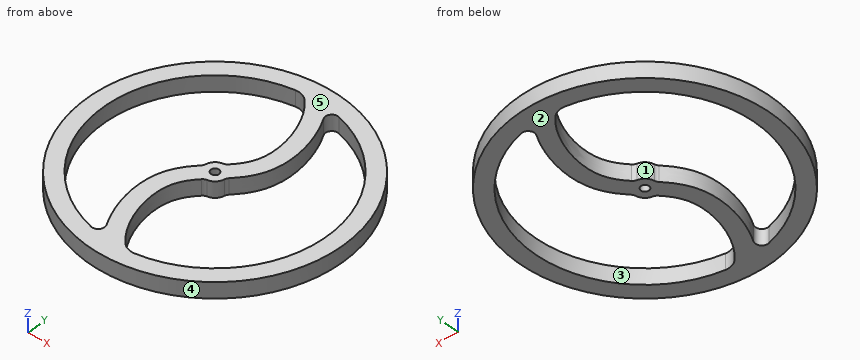
```python
from build123d import *

# Parameters (mm, degrees)
ESQUISSE1_R                  = 400
ESQUISSE1_R_2                = 350
BOSS_EXTRU_1_DEPTH           = 50
EXTRU_MINCE1_START           = -50
EXTRU_MINCE1_DEPTH           = 50
BOSS_EXTRU_2_START           = -50
BOSS_EXTRU_2_DEPTH           = 50
ENL_V_MAT_EXTRU_1_DEPTH      = 568.89083473
ENL_V_MAT_EXTRU_1_DEPTH_BACK = 568.89083473
ESQUISSE4_R                  = 12.5
ESQUISSE5_R                  = 35
ESQUISSE5_R_2                = 12.5
BOSS_EXTRU_3_DEPTH           = 50
CONG_2_R                     = 20


# Read off the part's stored shape, not the designer's step: Extru.-Mince1
with BuildPart() as part:
    # Esquisse1 → Boss.-Extru.1 (new body)
    with BuildSketch(Plane.XY):
        Circle(ESQUISSE1_R)
        Circle(ESQUISSE1_R_2, mode=Mode.SUBTRACT)
    extrude(amount=BOSS_EXTRU_1_DEPTH)

    # Extru.-Mince1 outline → Extru.-Mince1 (add)
    with BuildSketch(Plane.XY.offset(50).offset(EXTRU_MINCE1_START)):
        with BuildLine():
            add(Edge.make_bspline(
                [(-17.578582702, 332.223795956), (-13.006029397, 327.702076571), (-8.525799104, 322.703406145), (0.139661855, 311.878345733), (4.324902329, 306.052383763), (12.306325082, 293.716264205), (16.102617705, 287.206307092), (23.226392886, 273.652542218), (26.553972592, 266.608809401), (35.730163441, 244.906938456), (40.768636512, 229.677168598), (46.367738516, 206.627670241), (47.908578076, 198.910612565), (50.294392784, 183.568496034), (51.139268661, 175.94345939), (52.098340216, 160.947531132), (52.21238025, 153.576755976), (51.68889352, 139.252087771), (51.051205988, 132.298518999), (49.529565248, 122.298741474), (48.928334221, 119.037172715), (47.539683848, 112.675350651), (46.752582578, 109.576215008), (44.114742474, 100.538037841), (41.977452484, 94.806766085), (36.834878855, 83.551557811), (33.826996348, 78.025173728), (26.773354915, 66.867395642), (22.725430524, 61.236927426), (13.447578047, 49.660158587), (8.217643624, 43.715682454), (-3.507548172, 31.349570896), (-10.001973073, 24.928879975), (-24.829724062, 10.949936653), (-31.984427814, 3.887364914), (-45.291841947, -10.147456059), (-51.445384798, -17.120649798), (-62.760428782, -31.239396452), (-67.921923577, -38.386773856), (-77.204655719, -53.070631299), (-81.323727601, -60.608037124), (-88.444191242, -76.192121488), (-91.442984134, -84.236352462), (-95.084809692, -96.714540413), (-96.153499672, -100.931355257), (-98.014122409, -109.455423671), (-98.80637413, -113.763724761), (-100.790556161, -126.803188246), (-101.590583179, -135.648622106), (-102.243982659, -153.528217171), (-102.097194354, -162.562702654), (-100.936524717, -180.710794438), (-99.922487739, -189.824517197), (-97.092850599, -208.020658997), (-95.277151165, -217.103100248), (-88.710884536, -244.134069098), (-82.844776318, -261.867237944), (-72.075342178, -287.337160454), (-68.156254712, -295.638589688), (-59.690902904, -311.744851476), (-55.14473571, -319.549758973), (-45.517052393, -334.430345572), (-40.444476295, -341.515238116), (-35.080643578, -348.237488571)],
                knots=[0, 0, 0, 0, 0.0625, 0.0625, 0.125, 0.125, 0.1875, 0.1875, 0.25, 0.25, 0.375, 0.375, 0.4375, 0.4375, 0.5, 0.5, 0.5625, 0.5625, 0.625, 0.625, 0.65625, 0.65625, 0.6875, 0.6875, 0.75, 0.75, 0.8125, 0.8125, 0.875, 0.875, 0.9375, 0.9375, 1, 1, 1.06716091, 1.06716091, 1.134321821, 1.134321821, 1.201482731, 1.201482731, 1.268643642, 1.268643642, 1.335804552, 1.335804552, 1.369385007, 1.369385007, 1.402965463, 1.402965463, 1.470126373, 1.470126373, 1.537287283, 1.537287283, 1.604448194, 1.604448194, 1.671609104, 1.671609104, 1.805930925, 1.805930925, 1.873091836, 1.873091836, 1.940252746, 1.940252746, 2.00642831, 2.00642831, 2.00642831, 2.00642831], degree=3))
            ThreePointArc((-35.080643578, -348.237488571), (-17.562445732, -349.559094432), (0, -350))
            Line((0, -350), (17.578582702, -332.223795956))
            add(Edge.make_bspline(
                [(17.578582702, -332.223795956), (13.006029397, -327.702076571), (8.525799104, -322.703406145), (-0.139661855, -311.878345733), (-4.324902329, -306.052383763), (-12.306325082, -293.716264205), (-16.102617705, -287.206307092), (-23.226392886, -273.652542218), (-26.553972592, -266.608809401), (-35.730163441, -244.906938456), (-40.768636512, -229.677168598), (-46.367738516, -206.627670241), (-47.908578076, -198.910612565), (-50.294392784, -183.568496034), (-51.139268661, -175.94345939), (-52.098340216, -160.947531132), (-52.21238025, -153.576755976), (-51.68889352, -139.252087771), (-51.051205988, -132.298518999), (-49.529565248, -122.298741474), (-48.928334221, -119.037172715), (-47.539683848, -112.675350651), (-46.752582578, -109.576215008), (-44.114742474, -100.538037841), (-41.977452484, -94.806766085), (-36.834878855, -83.551557811), (-33.826996348, -78.025173728), (-26.773354915, -66.867395642), (-22.725430524, -61.236927426), (-13.447578047, -49.660158587), (-8.217643624, -43.715682454), (3.507548172, -31.349570896), (10.001973073, -24.928879975), (24.829724062, -10.949936653), (31.984427814, -3.887364914), (45.291841947, 10.147456059), (51.445384798, 17.120649798), (62.760428782, 31.239396452), (67.921923577, 38.386773856), (77.204655719, 53.070631299), (81.323727601, 60.608037124), (88.444191242, 76.192121488), (91.442984134, 84.236352462), (95.084809692, 96.714540413), (96.153499672, 100.931355257), (98.014122409, 109.455423671), (98.80637413, 113.763724761), (100.790556161, 126.803188246), (101.590583179, 135.648622106), (102.243982659, 153.528217171), (102.097194354, 162.562702654), (100.936524717, 180.710794438), (99.922487739, 189.824517197), (97.092850599, 208.020658997), (95.277151165, 217.103100248), (88.710884536, 244.134069098), (82.844776318, 261.867237944), (72.075342178, 287.337160454), (68.156254712, 295.638589688), (59.690902904, 311.744851476), (55.14473571, 319.549758973), (45.517052393, 334.430345572), (40.444476295, 341.515238116), (35.080643578, 348.237488571)],
                knots=[0, 0, 0, 0, 0.0625, 0.0625, 0.125, 0.125, 0.1875, 0.1875, 0.25, 0.25, 0.375, 0.375, 0.4375, 0.4375, 0.5, 0.5, 0.5625, 0.5625, 0.625, 0.625, 0.65625, 0.65625, 0.6875, 0.6875, 0.75, 0.75, 0.8125, 0.8125, 0.875, 0.875, 0.9375, 0.9375, 1, 1, 1.06716091, 1.06716091, 1.134321821, 1.134321821, 1.201482731, 1.201482731, 1.268643642, 1.268643642, 1.335804552, 1.335804552, 1.369385007, 1.369385007, 1.402965463, 1.402965463, 1.470126373, 1.470126373, 1.537287283, 1.537287283, 1.604448194, 1.604448194, 1.671609104, 1.671609104, 1.805930925, 1.805930925, 1.873091836, 1.873091836, 1.940252746, 1.940252746, 2.00642831, 2.00642831, 2.00642831, 2.00642831], degree=3))
            ThreePointArc((35.080643578, 348.237488571), (17.562445732, 349.559094432), (0, 350))
            Line((0, 350), (-17.578582702, 332.223795956))
        make_face()
    extrude(amount=EXTRU_MINCE1_DEPTH)

    # Esquisse3 → Boss.-Extru.2 (add)
    with BuildSketch(Plane.XY.offset(50).offset(BOSS_EXTRU_2_START)):
        with BuildLine():
            Line((-17.578582702, 332.223795956), (0, 350))
            ThreePointArc((0, 350), (-29.266098764, 348.774275805), (-58.327213726, 345.105688361))
            ThreePointArc((-58.327213726, 345.105688361), (-36.398453128, 343.581838752), (-17.578582702, 332.223795956))
        make_face()
        with BuildLine():
            Line((17.578582702, -332.223795956), (0, -350))
            ThreePointArc((0, -350), (29.266098764, -348.774275805), (58.327213726, -345.105688361))
            ThreePointArc((58.327213726, -345.105688361), (36.398453128, -343.581838752), (17.578582702, -332.223795956))
        make_face()
    extrude(amount=BOSS_EXTRU_2_DEPTH)

    # Esquisse4 → Enlèv. mat.-Extru.1 (cut, two sides: drawn at the far end of the back side and taken through both)
    with BuildSketch(Plane.XY.offset(50).offset(-ENL_V_MAT_EXTRU_1_DEPTH_BACK)):
        Circle(ESQUISSE4_R)
    extrude(amount=ENL_V_MAT_EXTRU_1_DEPTH + ENL_V_MAT_EXTRU_1_DEPTH_BACK, mode=Mode.SUBTRACT)

    # Esquisse5 → Boss.-Extru.3 (add)
    with BuildSketch(Plane.XY.offset(50)):
        Circle(ESQUISSE5_R)
        Circle(ESQUISSE5_R_2, mode=Mode.SUBTRACT)
    extrude(amount=-BOSS_EXTRU_3_DEPTH)

    # Congé2
    cong_2_edges = [part.edges().sort_by_distance(p)[0] for p in [
        (35.080643578, 348.237488571, 25),
        (-35.080643578, -348.237488571, 25),
        (34.993639035, -0.667253389, 25),
        (0.068739934, -34.999932497, 25),
        (-0.068739934, 34.999932497, 25),
        (-34.993639035, 0.667253389, 25),
    ]]
    fillet(cong_2_edges, radius=CONG_2_R)


solid = part.part
```
Verification items for the finished model (mm, model axes). Face numbers are marked on the shaded views. A direction names the side the tool comes from. Coordinates: 2 decimals unless noted, no trailing zeros. Return JSON: item names as keys, results as strings.
(1) Access from +Z, -Z, +X, -X, +Y, -Y to the whole of each face (thin tool, end or side, straight path). Record for the marked faces 1 and 2.
Filled sheet:
{"face 1": "+Z, -Z", "face 2": "-Z, +X, -X, +Y, -Y"}
(2) Section check A-A, the plane z = 25. Give the number of separate pieces and of enclosed holes in the cut face, and give its area (3 significant figures).
Filled sheet:
{"separate pieces": "1", "enclosed holes": "3", "area": "158,000 mm^2"}
(3) Thickness scan on line 1 along Y through (x, z) = (0, 20); line 2 along X through (y, z) = (-209, 46); line 3 along X through (y, z) = (-267, 19.5). Record the ranges inside material, lowest first.
Filled sheet:
{"line 1": "y = -400 to -311.86, -36.56 to -12.5, 12.5 to 36.56, 311.86 to 400", "line 2": "x = -341.06 to -280.75, -96.78 to -45.74, 280.75 to 341.06", "line 3": "x = -297.84 to -226.3, -80.42 to -26.26, 226.3 to 297.84"}
(4) Go/stop test with flat-tipped pins: pin 1 (3 mm diameter, centred on x = -72.5, z = 35, fed in from +Y); pin 2 (1 mm diameter, centred on x = 78, z = 16.5, fed in from -Y); pin 3 (6 mm diameter, centred on y = 202, z = 45, fed in from +X). Record where each tip stops, or that it passes through.
Filled sheet:
{"pin 1": "stops at y = 393.65", "pin 2": "stops at y = -392.42", "pin 3": "stops at x = 346.99"}
(5) Mould release check, pull along X, two halves, no side actions. Record for the marked faces 3, 4 and 5: pulls with the +X half, pulls with the -X half, needs draft (parallel to the pull), parting line crosses it, or undercut.
Filled sheet:
{"face 3": "undercut", "face 4": "parting line crosses it", "face 5": "needs draft"}
